```python
from build123d import *

# Parameters (mm, degrees)
SKETCH_1_R      = 2.5
EXTRUDE_1_DEPTH = 25
SKETCH_2_R      = 4.2
EXTRUDE_2_DEPTH = 1.9
SKETCH_3_R      = 4.25
EXTRUDE_3_DEPTH = 2
FILLET_1_R      = 1


with BuildPart() as part:
    # 草图1 → 凸台-拉伸1 (new body)
    with BuildSketch(Plane(origin=(0, 0, 0), x_dir=(1, 0, 0), z_dir=(0, 1, 0))):
        with Locations(Location((0, 0, 0), (0, 0, 270))):
            Circle(SKETCH_1_R)
    extrude(amount=EXTRUDE_1_DEPTH)

    # 草图2 → 凸台-拉伸2 (add)
    with BuildSketch(Plane(origin=(0, 25, 0), x_dir=(1, 0, 0), z_dir=(0, 1, 0))):
        with Locations(Location((0, 0, 0), (0, 0, 90))):
            Circle(SKETCH_2_R)
        Polygon((0.933529185, 1.100843583), (-0.486593916, 1.358881781), (-1.420123101, 0.258038198), (-0.933529185, -1.100843583), (0.486593916, -1.358881781), (1.420123101, -0.258038198), align=None, mode=Mode.SUBTRACT)
    extrude(amount=EXTRUDE_2_DEPTH)

    # 草图3 → 凸台-拉伸3 (add)
    with BuildSketch(Plane.XZ):
        with Locations(Location((0, 0, 0), (0, 0, 270))):
            Circle(SKETCH_3_R)
        Polygon((0.831789315, 1.179601572), (-0.605670271, 1.310151463), (-1.437459585, 0.130549891), (-0.831789315, -1.179601572), (0.605670271, -1.310151463), (1.437459585, -0.130549891), align=None, mode=Mode.SUBTRACT)
    extrude(amount=EXTRUDE_3_DEPTH)

    # 圆角1
    fillet_1_edges = [part.edges().sort_by_distance(p)[0] for p in [
        (0, 26.9, 4.2),
        (0, -2, 4.25),
    ]]
    fillet(fillet_1_edges, radius=FILLET_1_R)


solid = part.part
```
Check sheet for the modelled part. Datum: model origin and axes. Units: mm. A direction names the side the tool comes from. Round coordinates to 2 decimals unless told otherwise and drop trailing zeros. Order: outer loops, then holes, each group sorted by start corner. A loop starts at its lowest first (then second) coordinate and runs counter-clockwise, first axis right, second up.
1) Mould release check, pull along Y, two halves, no side actions. Record for faces 4 (the flat face through (0.7, 26.9, -1.4)), 5 (the flat face through (1.18, 25.94, -0.41)), 6 (the flat face through (0, 0, 0)), 7 (the flat face through (-2, 0, -2)): +Y half, -Y half, draft (parallel to the pull), parting line (faces both ways), or undercut.
2) Go/stop test with flat-tipped pins: pin 1 Ø3 at (x, y) = (-1, 9) entering from +Z; pin 2 Ø4 at (y, z) = (16, 1) entering from -X; pin 3 Ø1 at (y, z) = (19.5, 1.5) entering from -X. Record where each tip stops, or that it passes through.
3) Tool access check on faces 1 (the flat face through (1.016, -0.986, -0.729)), 2 (the cylindrical face through (-2.44, 12.32, -0.54)), 3 (the flat face through (0.23, 25.94, -1.23)). Record the directions out of +Z, -Z, +X, -X, +Y, -Y that give a thin tool (end or side, any length) a straight path to the whole face; none if there is none.
4) Section check A-A (y = 1.5). Record the boundary of the cut face in (x, z), and give its area (3 significant figures).
5) Scan lines: line 1 (Y direction, x = 3.25, z = -2.25); line 2 (Y direction, x = 1, z = 3.75); line 3 (Y direction, x = 0, z = 0). Record each from-to range of solid material in increasing order.
6) Section check B-B (x = 0). Record the boundary of the cut face in (y, z).
Result:
1. face 4: +Y half
1. face 5: draft
1. face 6: -Y half
1. face 7: undercut
2. pin 1: stops at z = 2.5
2. pin 2: stops at x = -2.5
2. pin 3: stops at x = -2.29
3. face 1: -Y
3. face 2: none
3. face 3: +Y
4. outline: circle Ø5 at (0, 0)
4. area: 19.6 mm2
5. line 1: y = -1.71 to 0, 25 to 26.56
5. line 2: y = -1.78 to 0, 25 to 26.63
5. line 3: y = 0 to 25
6. outline: (-2, -3.25) arc R1 ccw to (-1, -4.25) - (0, -4.25) - (0, -2.5) - (25, -2.5) - (25, -4.2) - (25.9, -4.2) arc R1 ccw to (26.9, -3.2) - (26.9, -1.27) - (25, -1.27) - (25, 1.27) - (26.9, 1.27) - (26.9, 3.2) arc R1 ccw to (25.9, 4.2) - (25, 4.2) - (25, 2.5) - (0, 2.5) - (0, 4.25) - (-1, 4.25) arc R1 ccw to (-2, 3.25) - (-2, 1.26) - (0, 1.26) - (0, -1.26) - (-2, -1.26) - close
